The drawing under review shows one solid part. Ordinate dimensions are in mm from its lowest x, y, z. A direction names the side the tool comes from. Coordinates: 2 decimals unless noted, no trailing zeros. Order: outer loops, then holes, each group sorted by start corner. A loop starts at its lowest first (then second) coordinate and runs counter-clockwise, first axis right, second up. Notation, with made-up numbers: (86.25, 51) -> (118.25, 51) arc R23 cw to (118.25, 85) -> close; hole circle Ø4 at (-9, 36). An arc over 180 degrees is marked (long way). Use one line per item in the form item = value.
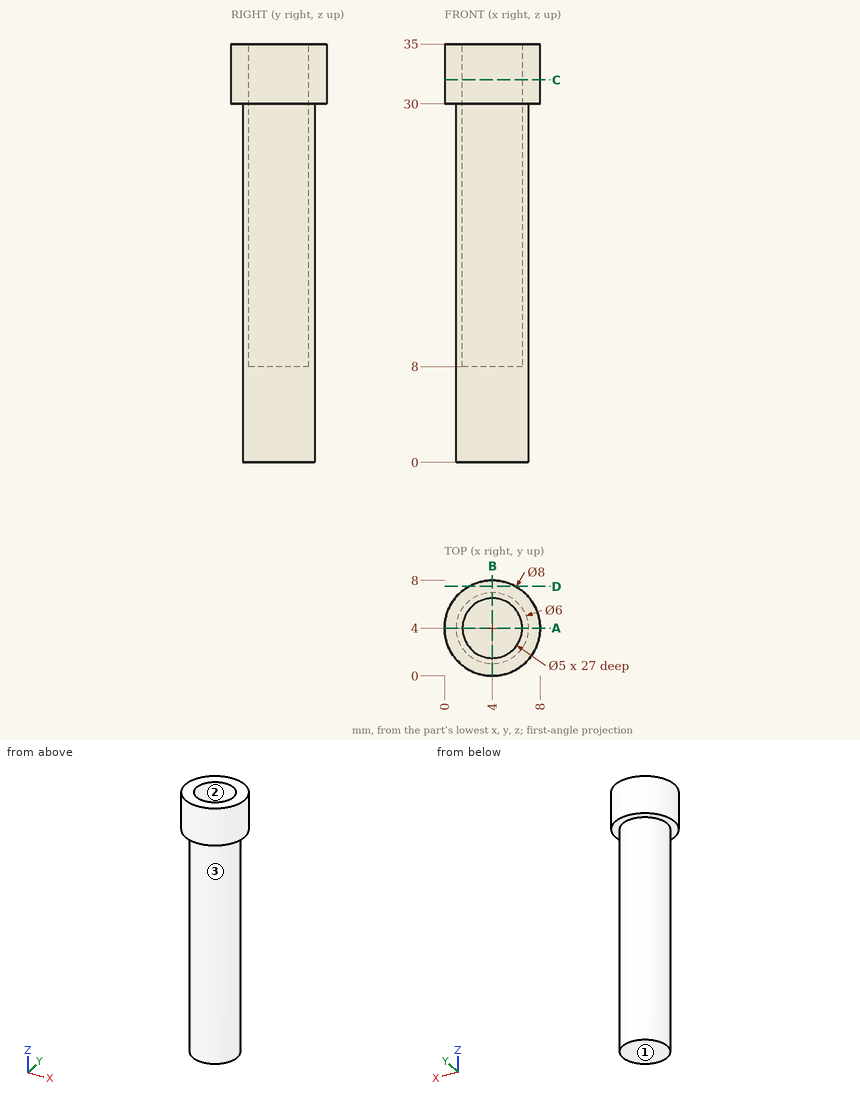
Item 1: To check wall thickness, follow L1, parallel to Y at x = 4, z = 18; L2, parallel to X at y = 3.25, z = 9.5; L3, parallel to Z at x = 1.25, y = 1.25. State the ranges of each line that lie inside material, in increasing order. Write a range as from..to.
Results found:
L1 = 1..1.5, 6.5..7
L2 = 1.1..1.62, 6.38..6.9
L3 = 30..35
Item 2: We need section A-A (y = 4). Write out the cut boundary in (x, z), plus the area to 3 significant figures.
Results found:
outline = (0, 30) -> (1, 30) -> (1, 0) -> (7, 0) -> (7, 30) -> (8, 30) -> (8, 35) -> (6.5, 35) -> (6.5, 8) -> (1.5, 8) -> (1.5, 35) -> (0, 35) -> close
area = 85.0 mm²
Item 3: We need section C-C (z = 32). Write out the cut boundary in (x, y).
Results found:
outline = circle Ø8 at (4, 4); hole circle Ø5 at (4, 4)
Item 4: Tool access review of the marked faces 1, 2 and 3: name each direction out of +Z, -Z, +X, -X, +Y, -Y from which nothing blocks a thin tool from reaching the whole face with its end or side.
Results found:
face_1 = -Z, +X, -X, +Y, -Y
face_2 = +Z
face_3 = -Z
Item 5: Clearance check with flat-ended pins moving along their axes: pin 1 (4 mm diameter, centred on x = 4, y = 4, fed in from +Z); pin 2 (1.5 mm diameter, centred on x = 3, z = 12, fed in from +Y); pin 3 (4 mm diameter, centred on y = 2.5, z = 27, fed in from -X). State where each tip first meets the part, or that it passes through.
Results found:
pin_1 = 8
pin_2 = 6.99
pin_3 = 1
Item 6: We need section D-D (y = 7.5). Write out the cut boundary in (x, z).
Results found:
outline = (2.06, 30) -> (5.94, 30) -> (5.94, 35) -> (2.06, 35) -> close
